Verification items for this drawing (mm, ordinates from the low corner). A direction names the side the tool comes from. Round coordinates to 2 decimals unless told otherwise and drop trailing zeros. Loops run counter-clockwise (first coordinate to the right, second up) from the corner with the lowest first, then second, coordinate; pieces in that order, holes last. Notation, with made-up numbers: (8, 13) -> (37, 13) arc R6 ccw to (37, 24) -> close; hole circle Ø11 at (-31, 83). An arc over 180 degrees is marked (long way). One line per item, written item: value. Start each with the question number.
1. Material ranges on L1, parallel to Y at x = 4.5, z = 46; L2, parallel to X at y = 5.5, z = 38.5; L3, parallel to Z at x = 5, y = 7.75, recorded low to high.
2. Set-up check for the marked faces 1 and 2: record each of +Z, -Z, +X, -X, +Y, -Y from which the full face is reachable in a straight line by a thin tool's end or side.
3. Cross-section at C-C on z = 21.5. Record the cut outline in (x, y).
4. Go/stop test with flat-tipped pins: pin 1 (1 mm diameter, centred on x = 2, z = 11, fed in from -Y); pin 2 (1 mm diameter, centred on y = 4, z = 8, fed in from -X); pin 3 (4 mm diameter, centred on y = 2.5, z = 20, fed in from +X); pin 4 (5 mm diameter, centred on x = 4, y = 5.5, fed in from -Z). Record where each tip stops, or that it passes through.
5. Cross-section at A-A on y = 4.5. Record the cut outline in (x, z), then the cut area to 3 significant figures.
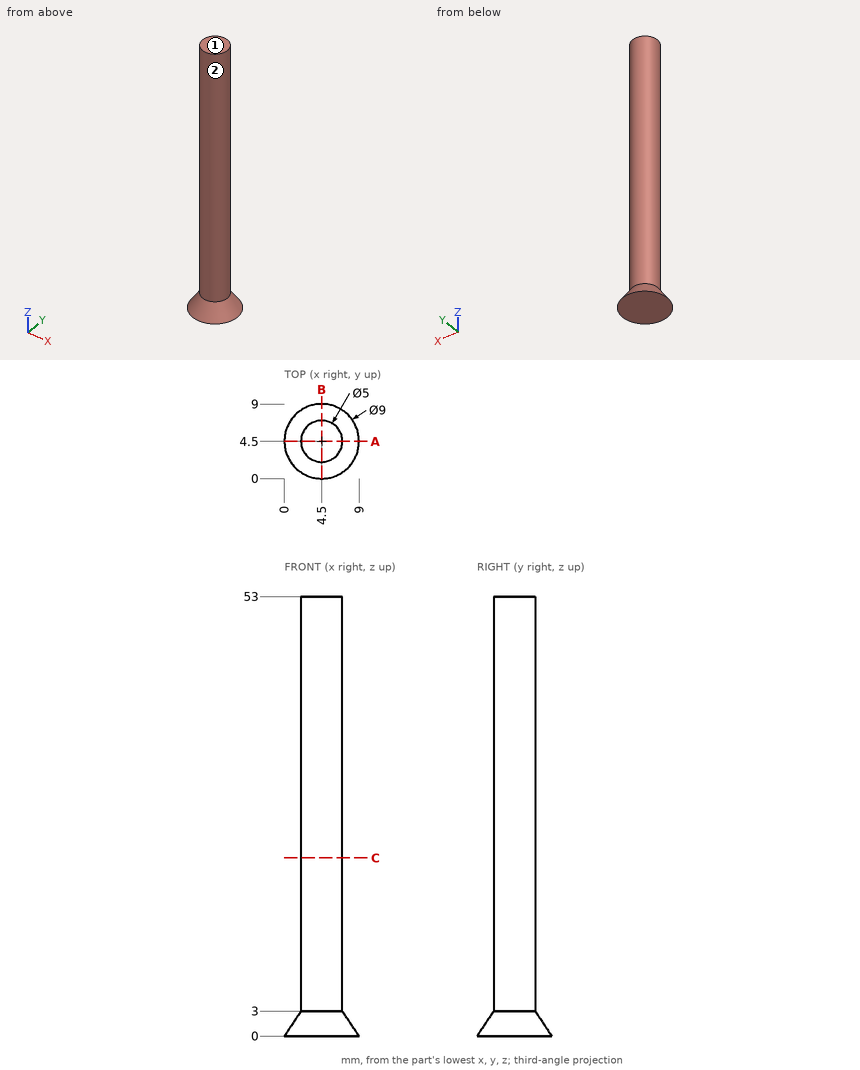
Taken from the geometry:
1. L1: y = 2 to 7
1. L2: x = 2.21 to 6.79
1. L3: z = 0 to 1.82
2. face 1: +Z, +X, -X, +Y, -Y
2. face 2: +Z
3. outline: circle Ø5 at (4.5, 4.5)
4. pin 1: stops at y = 3
4. pin 2: stops at x = 2
4. pin 3: stops at x = 7
4. pin 4: stops at z = 0
5. outline: (0, 0) -> (9, 0) -> (7, 3) -> (7, 53) -> (2, 53) -> (2, 3) -> close
5. area: 271 mm2
